from build123d import *

# Parameters (mm, degrees)
EXTRUDE_THIN1_DEPTH = 15
FILLET1_R           = 10
SKETCH2_R           = 2.5
CUT_EXTRUDE1_DEPTH  = 55
BOSS_EXTRUDE1_DEPTH = 30


with BuildPart() as part:
    # Sketch1 → Extrude-Thin1 (new, symmetric)
    with BuildSketch(Plane.XY):
        Polygon((-23.321428571, 30), (-23.321428571, -1.5), (27.678571429, -1.5), (27.678571429, 30), (24.678571429, 30), (24.678571429, 1.5), (-20.321428571, 1.5), (-20.321428571, 30), align=None)
    extrude(amount=EXTRUDE_THIN1_DEPTH, both=True)

    # Fillet1
    fillet1_edges = [part.edges().sort_by_distance(p)[0] for p in [
        (-21.821428571, 30, 15),
        (26.178571429, 30, 15),
        (-21.821428571, 30, -15),
        (26.178571429, 30, -15),
    ]]
    fillet(fillet1_edges, radius=FILLET1_R)

    # Sketch2 → Cut-Extrude1 (cut)
    with BuildSketch(Plane(origin=(27.678571429, 0, 0), x_dir=(0, 0, -1), z_dir=(1, 0, 0))):
        with Locations((0, 18.5)):
            Circle(SKETCH2_R)
    extrude(amount=-CUT_EXTRUDE1_DEPTH, mode=Mode.SUBTRACT)

    # Sketch4 → Boss-Extrude1 (add)
    with BuildSketch(Plane(origin=(0, 0, -15), x_dir=(-1, 0, 0), z_dir=(0, 0, -1))):
        Polygon((23.321428571, -1.5), (23.321428571, -43.5), (11.065130386, -43.5), (11.065130386, -41.079631184), (19.153220087, -41.079631184), (19.153220087, -1.5), align=None)
    extrude(amount=-BOSS_EXTRUDE1_DEPTH)


solid = part.part
Model file for the job. Use its own axes, mm. A direction names the side the tool comes from. Coordinates: 2 decimals unless noted, no trailing zeros. Write each loop counter-clockwise with the first axis right and the second up, starting at its lowest first coordinate (ties: lowest second). Pieces come first, ordered by that corner, then holes. Notation, with made-up numbers: (45.25, -1) -> (90.25, -1) arc R23 cw to (90.25, 30) -> close; hole circle Ø8 at (1.25, -33). An arc over 180 degrees is marked (long way). One line per item, written item: value. Start each with the question number.
1) Slice it at C-C on z = 0. Write the cut outline in (x, y).
2) Slice it at D-D on z = -7.5. Write the cut outline in (x, y).
3) Pull direction Y, two halves, no side cores. Call faces 6 (the face through (-17, -43.5, 0)), 7 (the face through (26.16, 27.15, -11.99)), 8 (the face through (-22, 21, 0)), 9 (the face through (-7, 0, -15)): +Y half, -Y half, draft (parallel to the pull), parting line (faces both ways), or undercut.
4) Slice it at A-A on y = 18.5. Write the cut outline in (x, z).
5) Which spindle directions (+Z, -Z, +X, -X, +Y, -Y) get a long thin tool onto all of the face, cutting with end or side? Do faces 1 (the face through (-23.321, -6, 0)), 2 (the face through (26, 21, 0)), 3 (the face through (4, -1.5, 0)), 4 (the face through (-11.065, -42, 0)), 5 (the face through (24.679, 13, 0)). Say none if no direction does.
6) Flat gauge pins, fed straight in: pin 1 Ø0.7 at (y, z) = (-43, 4.5) entering from +X; pin 2 Ø6 at (x, z) = (16.5, 3) entering from -Y; pin 3 Ø3 at (x, y) = (-12.5, -3.5) entering from +Z; pin 4 Ø6.5 at (y, z) = (18.5, 0) entering from +X. Where does each tip first touch, or does it go through?
7) Probe probe 1 along Y at (x, z) = (-14, 8.5); probe 2 along Y at (x, z) = (-21.4, 0); probe 3 along X at (y, z) = (25.5, -4.5). List the from-to ranges inside material, lowest first.
8) Slice it at B-B on x = -13. Write the cut outline in (y, z), then the cut area to 3 significant figures.
Answers follow:
1. outline: (-23.32, -43.5) -> (-11.07, -43.5) -> (-11.07, -41.08) -> (-19.15, -41.08) -> (-19.15, -1.5) -> (27.68, -1.5) -> (27.68, 16) -> (24.68, 16) -> (24.68, 1.5) -> (-20.32, 1.5) -> (-20.32, 16) -> (-23.32, 16) -> close; (-23.32, 21) -> (-20.32, 21) -> (-20.32, 30) -> (-23.32, 30) -> close; (24.68, 21) -> (27.68, 21) -> (27.68, 30) -> (24.68, 30) -> close
2. outline: (-23.32, -43.5) -> (-11.07, -43.5) -> (-11.07, -41.08) -> (-19.15, -41.08) -> (-19.15, -1.5) -> (27.68, -1.5) -> (27.68, 29.68) -> (24.68, 29.68) -> (24.68, 1.5) -> (-20.32, 1.5) -> (-20.32, 29.68) -> (-23.32, 29.68) -> close
3. face 6: -Y half
3. face 7: +Y half
3. face 8: undercut
3. face 9: draft
4. outline: (-23.32, -15) -> (-20.32, -15) -> (-20.32, -2.5) -> (-23.32, -2.5) -> close; (-23.32, 2.5) -> (-20.32, 2.5) -> (-20.32, 15) -> (-23.32, 15) -> close; (24.68, -15) -> (27.68, -15) -> (27.68, -2.5) -> (24.68, -2.5) -> close; (24.68, 2.5) -> (27.68, 2.5) -> (27.68, 15) -> (24.68, 15) -> close
5. face 1: +Z, -Z, -X, +Y, -Y
5. face 2: +X, -X
5. face 3: +Z, -Z, +X
5. face 4: +Z, -Z, +X, -Y
5. face 5: +Z, -Z, +Y
6. pin 1: x = -11.07
6. pin 2: y = -1.5
6. pin 3: through
6. pin 4: x = 27.68
7. probe 1: -43.5 to -41.08, -1.5 to 1.5
7. probe 2: -43.5 to 16, 21 to 30
7. probe 3: -23.32 to -20.32, 24.68 to 27.68
8. outline: (-43.5, -15) -> (-41.08, -15) -> (-41.08, 15) -> (-43.5, 15) -> close; (-1.5, -15) -> (1.5, -15) -> (1.5, 15) -> (-1.5, 15) -> close
8. area: 163 mm2
